```python
from build123d import *

# Parameters (mm, degrees)
SKETCH1_R           = 8
BOSS_EXTRUDE1_DEPTH = 10
SKETCH1_3_R         = 21.0025
BOSS_EXTRUDE2_DEPTH = 3.15
CUT_EXTRUDE1_DEPTH  = 4
SKETCH3_W           = 36.5
SKETCH3_H           = 19.8
CUT_EXTRUDE2_DEPTH  = 3
SKETCH4_W           = 7
SKETCH4_H           = 8.9
SKETCH4_R           = 1.375
BOSS_EXTRUDE3_DEPTH = 4.3
BOSS_EXTRUDE4_DEPTH = 3.15
CUT_EXTRUDE4_DEPTH  = 1.95
SKETCH9_R           = 21.0025
SKETCH9_R_2         = 8
BOSS_EXTRUDE8_DEPTH = 0.55
SKETCH10_R          = 8
CUT_EXTRUDE5_DEPTH  = 0.55
SKETCH11_W          = 7
SKETCH11_H          = 8.9
SKETCH11_R          = 1.375
CUT_EXTRUDE6_DEPTH  = 0.55


with BuildPart() as part:
    # Sketch1 → Boss-Extrude1 (new body)
    with BuildSketch(Plane(origin=(0, 0, 0), x_dir=(1, 0, 0), z_dir=(0, 1, 0))):
        with BuildLine():
            ThreePointArc((-11.637761812, 23.25), (-26, 0), (-11.637761812, -23.25))
            Line((-11.637761812, -23.25), (11.637761812, -23.25))
            ThreePointArc((11.637761812, -23.25), (26, 0), (11.637761812, 23.25))
            Line((11.637761812, 23.25), (-11.637761812, 23.25))
        make_face()
        Circle(SKETCH1_R, mode=Mode.SUBTRACT)
        with BuildLine():
            ThreePointArc((-3, -15.5), (0, -12.5), (3, -15.5))
            Line((3, -15.5), (3, -17))
            ThreePointArc((3, -17), (0, -20), (-3, -17))
            Line((-3, -17), (-3, -15.5))
        make_face(mode=Mode.SUBTRACT)
    extrude(amount=BOSS_EXTRUDE1_DEPTH)

    # Sketch1_3 → Boss-Extrude2 (add)
    with BuildSketch(Plane(origin=(0, 0, 0), x_dir=(1, 0, 0), z_dir=(0, 1, 0))):
        with BuildLine():
            Line((-5.874521255, -22.239716866), (-5.874521255, -23.25))
            Line((-5.874521255, -23.25), (5.874521255, -23.25))
            Line((5.874521255, -23.25), (5.874521255, -22.239716866))
            ThreePointArc((5.874521255, -22.239716866), (0, 23.0025), (-5.874521255, -22.239716866))
        make_face()
        Circle(SKETCH1_3_R, mode=Mode.SUBTRACT)
    extrude(amount=-BOSS_EXTRUDE2_DEPTH)

    # Sketch2 → Cut-Extrude1 (cut)
    with BuildSketch(Plane(origin=(0, 10, 0), x_dir=(1, 0, 0), z_dir=(0, 1, 0))):
        with BuildLine():
            Line((-18.15, -9.9), (-18.15, -18.616592062))
            ThreePointArc((-18.15, -18.616592062), (-16.556172611, -20.047272844), (-14.85, -21.341918845))
            Line((-14.85, -21.341918845), (-14.85, -11.9))
            Line((-14.85, -11.9), (14.85, -11.9))
            Line((14.85, -11.9), (14.85, -21.341918845))
            ThreePointArc((14.85, -21.341918845), (16.556172611, -20.047272844), (18.15, -18.616592062))
            Line((18.15, -18.616592062), (18.15, -9.9))
            Line((18.15, -9.9), (-18.15, -9.9))
        make_face()
    extrude(amount=-CUT_EXTRUDE1_DEPTH, mode=Mode.SUBTRACT)

    # Sketch3 → Cut-Extrude2 (cut)
    with BuildSketch(Plane(origin=(0, 10, 0), x_dir=(1, 0, 0), z_dir=(0, 1, 0))):
        with Locations((-7.75, 0)):
            Rectangle(SKETCH3_W, SKETCH3_H)
    extrude(amount=-CUT_EXTRUDE2_DEPTH, mode=Mode.SUBTRACT)

    # Sketch4 → Boss-Extrude3 (add)
    with BuildSketch(Plane(origin=(0, 10, 0), x_dir=(1, 0, 0), z_dir=(0, 1, 0))):
        with Locations((14, 5.45)):
            Rectangle(SKETCH4_W, SKETCH4_H)
        with Locations((14, 5)):
            Circle(SKETCH4_R, mode=Mode.SUBTRACT)
        with Locations((14, -5.45)):
            Rectangle(SKETCH4_W, SKETCH4_H)
        with Locations((14, -5)):
            Circle(SKETCH4_R, mode=Mode.SUBTRACT)
    extrude(amount=BOSS_EXTRUDE3_DEPTH)

    # Sketch6 → Boss-Extrude4 (add)
    with BuildSketch(Plane.XZ):
        with BuildLine():
            Line((-5.874521255, -23.25), (5.874521255, -23.25))
            Line((5.874521255, -23.25), (5.874521255, -22.239716866))
            ThreePointArc((5.874521255, -22.239716866), (0, -23.0025), (-5.874521255, -22.239716866))
            Line((-5.874521255, -22.239716866), (-5.874521255, -23.25))
        make_face()
    extrude(amount=BOSS_EXTRUDE4_DEPTH)

    # Sketch8 → Cut-Extrude4 (cut)
    with BuildSketch(Plane.XZ):
        with BuildLine():
            Line((-11.637761812, -23.25), (-5.874521255, -23.25))
            Line((-5.874521255, -23.25), (-5.874521255, -22.239716866))
            ThreePointArc((-5.874521255, -22.239716866), (-23.0025, 0), (-5.874521255, 22.239716866))
            Line((-5.874521255, 22.239716866), (-5.874521255, 23.25))
            Line((-5.874521255, 23.25), (-11.637761812, 23.25))
            ThreePointArc((-11.637761812, 23.25), (-26, 0), (-11.637761812, -23.25))
        make_face()
        with BuildLine():
            Line((5.874521255, 23.25), (5.874521255, 22.239716866))
            ThreePointArc((5.874521255, 22.239716866), (23.0025, 0), (5.874521255, -22.239716866))
            Line((5.874521255, -22.239716866), (5.874521255, -23.25))
            Line((5.874521255, -23.25), (11.637761812, -23.25))
            ThreePointArc((11.637761812, -23.25), (26, 0), (11.637761812, 23.25))
            Line((11.637761812, 23.25), (5.874521255, 23.25))
        make_face()
    extrude(amount=-CUT_EXTRUDE4_DEPTH, mode=Mode.SUBTRACT)

    # Sketch9 → Boss-Extrude8 (add)
    with BuildSketch(Plane.XZ):
        Circle(SKETCH9_R)
        Circle(SKETCH9_R_2, mode=Mode.SUBTRACT)
        with BuildLine():
            Line((-3, 15.5), (-3, 17))
            ThreePointArc((-3, 17), (0, 20), (3, 17))
            Line((3, 17), (3, 15.5))
            ThreePointArc((3, 15.5), (0, 12.5), (-3, 15.5))
        make_face(mode=Mode.SUBTRACT)
    extrude(amount=BOSS_EXTRUDE8_DEPTH)

    # Sketch10 → Cut-Extrude5 (cut)
    with BuildSketch(Plane(origin=(0, 7, 0), x_dir=(1, 0, 0), z_dir=(0, 1, 0))):
        with BuildLine():
            Line((-24.041422587, -9.9), (-18.15, -9.9))
            Line((-18.15, -9.9), (10.5, -9.9))
            Line((10.5, -9.9), (10.5, 9.9))
            Line((10.5, 9.9), (-24.041422587, 9.9))
            ThreePointArc((-24.041422587, 9.9), (-26, 0), (-24.041422587, -9.9))
        make_face()
        Circle(SKETCH10_R, mode=Mode.SUBTRACT)
    extrude(amount=-CUT_EXTRUDE5_DEPTH, mode=Mode.SUBTRACT)

    # Sketch11 → Cut-Extrude6 (cut)
    with BuildSketch(Plane(origin=(0, 14.3, 0), x_dir=(1, 0, 0), z_dir=(0, 1, 0))):
        with Locations((14, -5.45)):
            Rectangle(SKETCH11_W, SKETCH11_H)
        with Locations((14, -5)):
            Circle(SKETCH11_R, mode=Mode.SUBTRACT)
        with Locations((14, 5.45)):
            Rectangle(SKETCH11_W, SKETCH11_H)
        with Locations((14, 5)):
            Circle(SKETCH11_R, mode=Mode.SUBTRACT)
    extrude(amount=-CUT_EXTRUDE6_DEPTH, mode=Mode.SUBTRACT)


solid = part.part
```
Work out the finished part from the listing and answer in its coordinate system (mm). A direction names the side the tool comes from. Round coordinates to 2 decimals unless told otherwise and drop trailing zeros. Loops run counter-clockwise (first coordinate to the right, second up) from the corner with the lowest first, then second, coordinate; pieces in that order, holes last.
(1) For faces 5 (the flat face through (14, 12, -1)), 6 (the flat face through (3, 5, 16)), 7 (the cylindrical face through (12.626, 11.849, -5.06)), determine the directions among +Z, -Z, +X, -X, +Y, -Y from which every point of the face is accessible in a straight line to the end or side of a thin tool.
Computed values:
face 5: +X, -X, +Y
face 6: +Y, -Y
face 7: +Y
(2) The mould has two halves that part along X. Classify faces 1 (the flat face through (17.5, 12, 6)), 2 (the cylindrical face through (0.1, 4.8, 12.5)), 3 (the flat face through (14, 12, -9.9)), 4 (the flat face through (10.5, 9, 0)): pulls with the +X half, pulls with the -X half, needs draft (parallel to the pull), parting line crosses it, or undercut.
Computed values:
face 1: pulls with the +X half
face 2: undercut
face 3: needs draft
face 4: pulls with the -X half
(3) The part is cut by section A-A, the plane x = -2. Give the vertices of the cut face in (y, z).
Computed values:
outline: (-3.15, -23.25) - (10, -23.25) - (10, -9.9) - (6.45, -9.9) - (6.45, -7.75) - (-0.55, -7.75) - (-0.55, -20.91) - (-3.15, -20.91) - close; (-3.15, 20.91) - (-0.55, 20.91) - (-0.55, 19.24) - (10, 19.24) - (10, 23.25) - (-3.15, 23.25) - close; (-0.55, 7.75) - (6.45, 7.75) - (6.45, 9.9) - (6, 9.9) - (6, 11.9) - (10, 11.9) - (10, 13.26) - (-0.55, 13.26) - close
(4) Find the intervals of material crossed by L1, parallel to Z at x = 14, y = 12.25 (3 decimals); L2, parallel to X at y = 12.2, z = -5 (3 decimals); L3, parallel to X at y = 2.5, z = 0, in increasing order.
Computed values:
L1: z = -9.9 to -6.375, -3.625 to -1, 1 to 3.625, 6.375 to 9.9
L2: x = 10.5 to 12.625, 15.375 to 17.5
L3: x = -26 to -8, 8 to 26
(5) The part is cut by section D-D, the plane x = -10.5. Give the vertices of the cut face in (y, z).
Computed values:
outline: (-3.15, -20.47) - (1.95, -20.47) - (1.95, -23.25) - (10, -23.25) - (10, -9.9) - (6.45, -9.9) - (6.45, 9.9) - (6, 9.9) - (6, 11.9) - (10, 11.9) - (10, 23.25) - (1.95, 23.25) - (1.95, 20.47) - (-3.15, 20.47) - (-3.15, 18.19) - (-0.55, 18.19) - (-0.55, -18.19) - (-3.15, -18.19) - close
(6) Each of these flat-tipped pins is pushed along its axis until it touches: P1, Ø4.5, axis at x = 14, z = -5, coming from the -Y side; P2, Ø10, axis at x = -5, z = 3.5, coming from the +Y side; P3, Ø12, axis at x = -3, z = -5, coming from the +Y side. Where does it stop, or does it pass through?
Computed values:
P1: stops at y = -0.55
P2: stops at y = 6.45
P3: stops at y = 10
